Print and shaded views of the part. All mm, measured from the part's lowest x, y and z. Give positions to 0.01 mm unless a question says otherwise; leave off trailing zeros. Loops run counter-clockwise (first coordinate to the right, second up) from the corner with the lowest first, then second, coordinate; pieces in that order, holes last. Notation, with made-up numbers: M 9.5,-28 L 40.5,-28 A5 ccw 40.5,-21 Z; hole C 18.25,-18 d10. An arc over 180 degrees is marked long. Put each result on its own line as item: value. Start each with the question number.
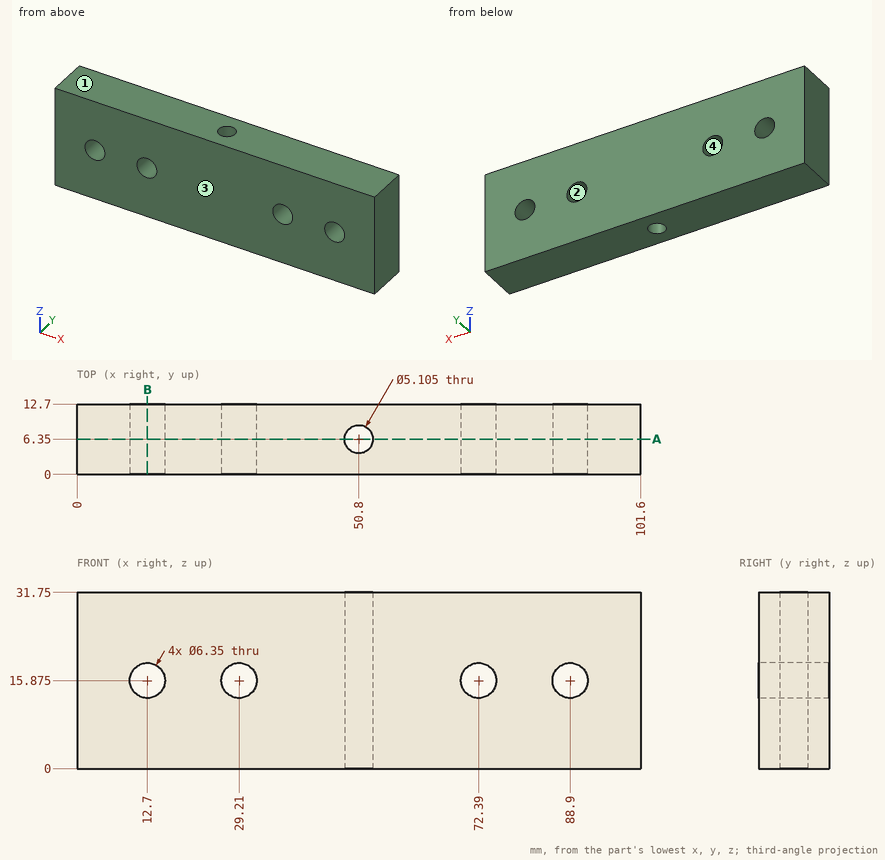
1) Wall check: L1, parallel to Z at x = 72.39, y = 6.25; L2, parallel to X at y = 7, z = 15; L3, parallel to X at y = 4, z = 29.5 (1 decimal). Give the ranges that are in metal, low to high.
2) Mould opens along Z. For the marked faces 1, 2, 3 and 4 say: +Z half, -Z half, draft (parallel to the pull), parting line (faces both ways), or undercut.
3) Pin check, flat tips, straight feed: pin 1 Ø4 at (x, z) = (88.9, 15.875) entering from -Y; pin 2 Ø6 at (x, y) = (50.8, 6.35) entering from +Z. Stop position of each tip, or through.
4) Band-saw the part on A-A on y = 6.35. State how many separate pieces and enclosed holes the cut face has, then the cut area to 3 significant figures.
5) Band-saw the part on B-B on x = 12.7. Give the cut face in (y, z).
Evaluation:
1. L1: 0 to 12.7, 19.05 to 31.75
1. L2: 0 to 9.65, 15.75 to 26.16, 32.26 to 48.33, 53.27 to 69.34, 75.44 to 85.85, 91.95 to 101.6
1. L3: 0 to 49.8, 51.8 to 101.6
2. face 1: +Z half
2. face 2: undercut
2. face 3: draft
2. face 4: undercut
3. pin 1: through
3. pin 2: z = 31.75
4. separate pieces: 2
4. enclosed holes: 4
4. area: 2,940 mm2
5. outline: M 0,0 L 12.7,0 L 12.7,12.7 L 0,12.7 Z; M 0,19.05 L 12.7,19.05 L 12.7,31.75 L 0,31.75 Z
